Check sheet for the modelled part. Datum: model origin and axes. Units: mm. A direction names the side the tool comes from. Coordinates: 2 decimals unless noted, no trailing zeros. Loops run counter-clockwise (first coordinate to the right, second up) from the corner with the lowest first, then second, coordinate; pieces in that order, holes last. Notation, with made-up numbers: (-18.5, -26) -> (37.5, -26) arc R14 cw to (37.5, -11) -> close; hole circle Ø2 at (61.25, 55.5). An arc over 180 degrees is marked (long way). Use CSV: the item, a comma, the result in double quotes.
```python
from build123d import *

# Parameters (mm, degrees)
F1_DEPTH = 152.4
F3_ANGLE = 92.3138340894
F4_DEPTH = 25.4


with BuildPart() as f1:
    # F0 (on Front) → F1 (new body)
    with BuildSketch(Plane.XZ):
        Polygon((3.175, -1.8330871047), (3.175, 1.8330871047), (0, 3.6661742094), (-3.175, 1.8330871047), (-3.175, -1.8330871047), (0, -3.6661742094), align=None)
    extrude(amount=F1_DEPTH)

    # F2 (on face) → F3 (revolve)
    with BuildSketch(Plane.XZ.offset(152.4)):
        Polygon((-3.175, 1.8330871047), (-3.175, -1.8330871047), (0, -3.6661742094), (3.175, -1.8330871047), (3.175, 1.8330871047), (0, 3.6661742094), align=None)
    revolve(axis=Axis((-9.525, -152.4, 0.9165435523), (0, 0, -1)), revolution_arc=F3_ANGLE)

    # F4 (add): a face of the model
    f4_faces = [f1.faces().sort_by_distance(p)[0] for p in [
        (-9.9095532751, -161.9172340403, 0),
    ]]
    extrude(f4_faces, amount=F4_DEPTH)


solid = f1.part
```
1) Go/stop test with flat-tipped pins: pin 1 Ø1.8 at (y, z) = (-65.5, 0) entering from -X (3 decimals); pin 2 Ø2 at (x, z) = (-20.5, -1) entering from +Y; pin 3 Ø10 at (x, y) = (-8, -127) entering from +Z. Record where each tip stops, or that it passes through.
Answer below:
pin 1,"stops at x = -3.175"
pin 2,"stops at y = -158.27"
pin 3,"stops at z = 1.93"
2) Cross-section at C-C on x = -24. Record the boundary of the cut face in (y, z).
Answer below:
outline,"(-164.53, -1.83) -> (-161.35, -3.67) -> (-158.17, -1.83) -> (-158.17, 1.83) -> (-161.35, 3.67) -> (-164.53, 1.83) -> close"
3) Draft check along X on faces 6 (the flat face through (1.57, -75.13, -2.76)), 7 (the cylindrical face through (-5.075, -156.93, -0.026)), 8 (the flat face through (-1.61, -75.133, -2.737)), 9 (the flat face through (0, 0, 0)). Enter one of: released by +X, released by -X, zero draft, split by the parting line, or undercut.
Answer below:
face 6,"released by +X"
face 7,"undercut"
face 8,"released by -X"
face 9,"zero draft"
4) Cross-section at B-B on y = -91. Record the boundary of the cut face in (x, z) (3 decimals), and give its area (3 significant figures).
Answer below:
outline,"(-3.175, -1.833) -> (0, -3.666) -> (3.175, -1.833) -> (3.175, 1.833) -> (0, 3.666) -> (-3.175, 1.833) -> close"
area,"34.9 mm²"
5) Thickness scan on line 1 along Y through (x, z) = (-9, -1.75); line 2 along X through (y, z) = (-34, -0.25) (3 decimals); line 3 along X through (y, z) = (-84, 3.25). Record the ranges inside material, lowest first. Write a range as from..to.
Answer below:
line 1,"y = -165.09..-158.73"
line 2,"x = -3.175..3.175"
line 3,"x = -0.72..0.72"
6) Access from +Z, -Z, +X, -X, +Y, -Y to the whole of each face (thin tool, end or side, straight path). Record for faces 1 (the flat face through (1.61, -75.133, 2.737)), 2 (the flat face through (-3.175, -75, 0)), 3 (the flat face through (3.175, -75, 0)), 4 (the flat face through (-22.29, -158.24, 0.03)), 5 (the flat face through (-1.57, -75.13, 2.76)).
Answer below:
face 1,"+Z, +X, +Y, -Y"
face 2,"+Z, -Z, -X, +Y"
face 3,"+Z, -Z, +X, +Y, -Y"
face 4,"+Z, -Z, +Y"
face 5,"+Z, -X, +Y"
7) Cross-section at A-A on z = -0.5. Record the boundary of the cut face in (x, y) (3 decimals), and give its area (3 significant figures).
Answer below:
outline,"(-35.417, -164.064) -> (-10.038, -165.09) arc R12.7 ccw to (3.175, -152.4) -> (3.175, 0) -> (-3.175, 0) -> (-3.175, -152.4) arc R6.35 cw to (-9.781, -158.745) -> (-35.161, -157.719) -> close"
area,"1,230 mm²"
